```python
from build123d import *

# Parameters (mm, degrees)
SKETCH1_R           = 1.27
SKETCH1_W           = 43.18
SKETCH1_H           = 20.32
BOSS_EXTRUDE1_DEPTH = 9.525
SKETCH2_R           = 1.7272
CUT_EXTRUDE1_DEPTH  = 12.7


with BuildPart() as part:
    # Sketch1 → Boss-Extrude1 (new body)
    with BuildSketch(Plane.XY):
        Polygon((0, 0), (63.5, 0), (63.5, 15.875), (76.2, 15.875), (76.2, 0), (101.6, 0), (101.6, 25.4), (0, 25.4), align=None)
        with Locations((3.048, 18.415)):
            Circle(SKETCH1_R, mode=Mode.SUBTRACT)
        with Locations((3.048, 5.715)):
            Circle(SKETCH1_R, mode=Mode.SUBTRACT)
        with Locations((52.832, 18.415)):
            Circle(SKETCH1_R, mode=Mode.SUBTRACT)
        with Locations((52.832, 5.715)):
            Circle(SKETCH1_R, mode=Mode.SUBTRACT)
        with Locations((27.94, 12.065)):
            Rectangle(SKETCH1_W, SKETCH1_H, mode=Mode.SUBTRACT)
    extrude(amount=BOSS_EXTRUDE1_DEPTH)

    # Sketch2 → Cut-Extrude1 (cut)
    with BuildSketch(Plane.XZ):
        with Locations((60.2488, 4.7625)):
            Circle(SKETCH2_R)
        with Locations((79.2988, 4.7625)):
            Circle(SKETCH2_R)
    extrude(amount=-CUT_EXTRUDE1_DEPTH, mode=Mode.SUBTRACT)


solid = part.part
```
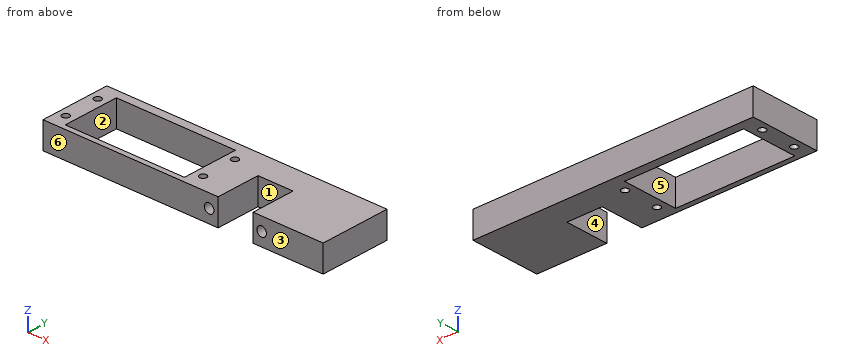
Read the model definition and answer for the solid it produces. Units are mm, in the model's axes. Face numbers are marked on the shaded views. A direction names the side the tool comes from. Round coordinates to 2 decimals unless told otherwise and drop trailing zeros. Loops run counter-clockwise (first coordinate to the right, second up) from the corner with the lowest first, then second, coordinate; pieces in that order, holes last. Notation, with made-up numbers: (55.5, 47.25) -> (99.5, 47.25) arc R32 cw to (99.5, 74.25) -> close; hole circle Ø9 at (13, 71). An arc over 180 degrees is marked (long way). One line per item, written item: value.
1) Consider L1, parallel to X at y = 9.5, z = 9; L2, parallel to Y at x = 19, z = 1 (3 decimals); L3, parallel to X at y = 18.5, z = 1. Determine where each line is inside the solid, lowest interval first. Write a range as [from, to].
Answer list:
L1: x = [0, 6.35], [49.53, 63.5], [76.2, 101.6]
L2: y = [0, 1.905], [22.225, 25.4]
L3: x = [0, 1.78], [4.32, 6.35], [49.53, 51.56], [54.1, 101.6]
2) The mould has two halves that part along Y. Classify the marked faces 4, 5 and 6: pulls with the +Y half, pulls with the -Y half, needs draft (parallel to the pull), parting line crosses it, or undercut.
Answer list:
face 4: needs draft
face 5: undercut
face 6: pulls with the -Y half
3) A flat-ended cylindrical pin translates along its axis: P1, Ø4, axis at x = 71, z = 6.5, coming from the -Y side (3 decimals). Find the tip coordinate at first contact, or state that the pin passes through.
Answer list:
P1: stops at y = 15.875
4) A cutting plane is placed at A-A (x = 46). Determine the outline of the cut face in (y, z) (3 decimals).
Answer list:
outline: (0, 0) -> (1.905, 0) -> (1.905, 9.525) -> (0, 9.525) -> close; (22.225, 0) -> (25.4, 0) -> (25.4, 9.525) -> (22.225, 9.525) -> close
5) A cutting plane is placed at C-C (z = 7.5). Determine the outline of the cut face in (x, y) (3 decimals), and give its area (3 significant figures).
Answer list:
outline: (0, 0) -> (63.5, 0) -> (63.5, 15.875) -> (76.2, 15.875) -> (76.2, 0) -> (101.6, 0) -> (101.6, 25.4) -> (0, 25.4) -> close; hole circle Ø2.54 at (3.048, 5.715); hole circle Ø2.54 at (3.048, 18.415); hole (6.35, 1.905) -> (49.53, 1.905) -> (49.53, 22.225) -> (6.35, 22.225) -> close; hole circle Ø2.54 at (52.832, 5.715); hole circle Ø2.54 at (52.832, 18.415)
area: 1,480 mm²
6) A cutting plane is placed at D-D (x = 66). Determine the outline of the cut face in (y, z) (3 decimals).
Answer list:
outline: (15.875, 0) -> (25.4, 0) -> (25.4, 9.525) -> (15.875, 9.525) -> close
7) A cutting plane is placed at B-B (y = 3). Give the number of separate pieces and of enclosed holes in the cut face, and give its area (3 significant figures).
Answer list:
separate pieces: 3
enclosed holes: 2
area: 417 mm²
8) For the marked faces 1, 2 and 3, determine the directions among +Z, -Z, +X, -X, +Y, -Y from which every point of the face is accessible in a straight line to the end or side of a thin tool.
Answer list:
face 1: +Z, -Z, -Y
face 2: +Z, -Z
face 3: +Z, -Z, +X, -X, -Y
